Verification items for the finished model (mm, model axes). A direction names the side the tool comes from. Give positions to 0.01 mm unless a question says otherwise; leave off trailing zeros. Order: outer loops, then holes, each group sorted by start corner. A loop starts at its lowest first (then second) coordinate and runs counter-clockwise, first axis right, second up.
(1) Access from +Z, -Z, +X, -X, +Y, -Y to the whole of each face (thin tool, end or side, straight path). Record for faces 1 (the face through (9.525, 0, -33)), 2 (the face through (-12.55, 5.617, 12.103)).
(2) Sectioned sample at B-B on z = -22. Record the cut outline in (x, y), plus the area to 3 significant figures.
(3) Scan lines: L1, parallel to X at y = 2.25, z = 13.44; L2, parallel to Z at x = 11.5, y = 4.5 (3 decimals); L3, parallel to X at y = 4.25, z = -20.5. Record each from-to range of solid material in increasing order.
(4) Sectioned sample at C-C on y = -6.5. Record the cut outline in (x, z) (3 decimals), plus the area to 3 significant figures.
(5) Sectioned sample at A-A on x = 0. Record the cut outline in (y, z) (3 decimals), plus the area to 3 significant figures.
(6) Gauge pin test, flat ends, axial feed: pin 1 (8 mm diameter, centred on x = -1.5, z = -8, fed in from -Y); pin 2 (0.8 mm diameter, centred on x = -9, z = -33.5, fed in from -Y). Record the tip position at first contact, or that the pin passes through.
(7) Mould release check, pull along Z, two halves, no side actions. Record for faces 3 (the face through (-16.51, -1, 1)), 4 (the face through (-0.307, 1.267, 39.987)), 5 (the face through (0, 3, 41.275)): pulls with the +Z half, pulls with the -Z half, needs draft (parallel to the pull), parting line crosses it, or undercut.
```python
from build123d import *

# Parameters (mm, degrees)
SKETCH1_W           = 38.1
SKETCH1_H           = 82.55
BOSS_EXTRUDE1_DEPTH = 12.7
SHELL1_T            = -2.54
SKETCH2_R           = 13.97
CUT_EXTRUDE1_DEPTH  = 86.666183527
SKETCH3_R           = 1.7
CUT_EXTRUDE2_DEPTH  = 51.883275494
EXTRUDE_THIN1_START = 11.43
SKETCH4_R           = 2.97
SKETCH4_R_2         = 1.7
EXTRUDE_THIN1_DEPTH = 11.43
CUT_EXTRUDE3_DEPTH  = 2.54


with BuildPart() as part:
    # Sketch1 → Boss-Extrude1 (new, symmetric)
    with BuildSketch(Plane(origin=(0, 0, 0), x_dir=(1, 0, 0), z_dir=(0, 1, 0))):
        Rectangle(SKETCH1_W, SKETCH1_H)
    extrude(amount=BOSS_EXTRUDE1_DEPTH, both=True)

    # Shell1
    shell1_openings = [part.faces().sort_by_distance(p)[0] for p in [
        (0, -12.7, 0),
    ]]
    offset(amount=SHELL1_T, openings=shell1_openings, kind=Kind.INTERSECTION)

    # Sketch2 → Cut-Extrude1 (cut, through all)
    with BuildSketch(Plane(origin=(0, 0, -41.275), x_dir=(-1, 0, 0), z_dir=(0, 0, -1))):
        with Locations((0, -12.7)):
            Circle(SKETCH2_R)
    extrude(amount=-CUT_EXTRUDE1_DEPTH, mode=Mode.SUBTRACT)

    # Sketch3 → Cut-Extrude2 (cut, through all)
    with BuildSketch(Plane.XZ.offset(-10.16)):
        with Locations(Location((11.5, 13.44, 0), (0, 0, 270))):
            Circle(SKETCH3_R)
        with Locations(Location((11.5, -33.06, 0), (0, 0, 270))):
            Circle(SKETCH3_R)
        with Locations(Location((-11.5, -33.06, 0), (0, 0, 270))):
            Circle(SKETCH3_R)
        with Locations(Location((-11.5, 13.44, 0), (0, 0, 270))):
            Circle(SKETCH3_R)
    extrude(amount=-CUT_EXTRUDE2_DEPTH, mode=Mode.SUBTRACT)

    # Sketch4 → Extrude-Thin1 (add)
    # profile 1 of 4: a face of its own
    with BuildSketch(Plane.XZ.offset(-10.16).offset(EXTRUDE_THIN1_START)):
        with Locations((11.5, 13.44)):
            Circle(SKETCH4_R)
        with Locations((11.5, 13.44)):
            Circle(SKETCH4_R_2, mode=Mode.SUBTRACT)
    # profile 2 of 4: a face of its own
    with BuildSketch(Plane.XZ.offset(-10.16).offset(EXTRUDE_THIN1_START)):
        with Locations((-11.5, 13.44)):
            Circle(SKETCH4_R)
        with Locations((-11.5, 13.44)):
            Circle(SKETCH4_R_2, mode=Mode.SUBTRACT)
    # profile 3 of 4: a face of its own
    with BuildSketch(Plane.XZ.offset(-10.16).offset(EXTRUDE_THIN1_START)):
        with Locations((-11.5, -33.06)):
            Circle(SKETCH4_R)
        with Locations((-11.5, -33.06)):
            Circle(SKETCH4_R_2, mode=Mode.SUBTRACT)
    # profile 4 of 4: a face of its own
    with BuildSketch(Plane.XZ.offset(-10.16).offset(EXTRUDE_THIN1_START)):
        with Locations((11.5, -33.06)):
            Circle(SKETCH4_R)
        with Locations((11.5, -33.06)):
            Circle(SKETCH4_R_2, mode=Mode.SUBTRACT)
    extrude(amount=-EXTRUDE_THIN1_DEPTH)

    # Sketch5 → Cut-Extrude3 (cut)
    with BuildSketch(Plane.XZ.offset(1.27)):
        Polygon((-10.16, -15.94), (-9.525, -15.94), (-9.525, -36.83), (9.525, -36.83), (9.525, -15.94), (10.16, -15.94), (10.16, 15.94), (-10.16, 15.94), align=None)
    extrude(amount=-CUT_EXTRUDE3_DEPTH, mode=Mode.SUBTRACT)


solid = part.part
```
Ans:
1. face 1: -Y
1. face 2: +Y, -Y
2. outline: (-19.05, -12.7) - (-16.51, -12.7) - (-16.51, 10.16) - (16.51, 10.16) - (16.51, -12.7) - (19.05, -12.7) - (19.05, 12.7) - (-19.05, 12.7) - close
2. area: 213 mm2
3. L1: x = -19.05 to -16.51, -14.47 to -13.2, -9.8 to -8.53, 8.53 to 9.8, 13.2 to 14.47, 16.51 to 19.05
3. L2: z = -41.275 to -38.735, -36.03 to -34.76, -31.36 to -30.09, 10.47 to 11.74, 15.14 to 16.41, 38.735 to 41.275
3. L3: x = -19.05 to -16.51, 16.51 to 19.05
4. outline: (-19.05, -41.275) - (-12.519, -41.275) - (-12.519, -38.735) - (-16.51, -38.735) - (-16.51, 38.735) - (-12.519, 38.735) - (-12.519, 41.275) - (-19.05, 41.275) - close; (12.519, -41.275) - (19.05, -41.275) - (19.05, 41.275) - (12.519, 41.275) - (12.519, 38.735) - (16.51, 38.735) - (16.51, -38.735) - (12.519, -38.735) - close
4. area: 460 mm2
5. outline: (1.27, -41.275) - (12.7, -41.275) - (12.7, 41.275) - (1.27, 41.275) - (1.27, 38.735) - (10.16, 38.735) - (10.16, -38.735) - (1.27, -38.735) - close
5. area: 255 mm2
6. pin 1: stops at y = 10.16
6. pin 2: stops at y = 1.27
7. face 3: undercut
7. face 4: needs draft
7. face 5: pulls with the +Z half
